Build history of the part. All positions in model axes, mm. Face numbers are marked on the shaded views. A direction names the side the tool comes from. Give positions to 0.01 mm unless a question says otherwise; leave off trailing zeros. Order: outer loops, then holes, each group sorted by start corner. A loop starts at its lowest first (then second) coordinate and runs counter-clockwise, first axis right, second up. Notation, with made-up numbers: (1, 46) -> (23, 46) arc R27 ccw to (23, 76) -> close; hole circle Ø3 at (85.5, 47). An arc over 180 degrees is marked (long way). Use a Markdown table: item, result. Add a question column.
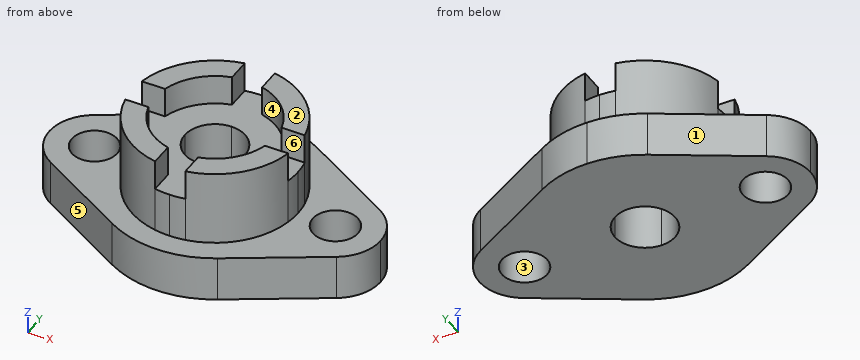
```python
from build123d import *

# Parameters (mm, degrees)
F1_DEPTH = 19.05
F2_DEPTH = 38.1
F3_DEPTH = 50.8


with BuildPart() as f1:
    # F0 (on Top) → F1 (new body)
    with BuildSketch(Plane.XY):
        with BuildLine():
            Line((41.275, 0), (34.925, 0))
            ThreePointArc((34.925, 0), (34.7791644937, -3.1883133656), (34.3428758988, -6.35))
            ThreePointArc((34.3428758988, -6.35), (24.6957043329, -24.6957043329), (6.35, -34.3428758988))
            ThreePointArc((6.35, -34.3428758988), (3.1883133656, -34.7791644937), (0, -34.925))
            ThreePointArc((0, -34.925), (-3.1883133656, -34.7791644937), (-6.35, -34.3428758988))
            ThreePointArc((-6.35, -34.3428758988), (-24.6957043329, -24.6957043329), (-34.3428758988, -6.35))
            ThreePointArc((-34.3428758988, -6.35), (-34.7791644937, -3.1883133656), (-34.925, 0))
            ThreePointArc((-34.925, 0), (-34.7791644937, 3.1883133656), (-34.3428758988, 6.35))
            ThreePointArc((-34.3428758988, 6.35), (-24.6957043329, 24.6957043329), (-6.35, 34.3428758988))
            ThreePointArc((-6.35, 34.3428758988), (-3.1883133656, 34.7791644937), (0, 34.925))
            Line((0, 34.925), (0, 44.45))
            ThreePointArc((0, 44.45), (-11.5045065548, 42.9354029785), (-22.225, 38.4948291982))
            Line((-22.225, 38.4948291982), (-60.325, 16.4977839421))
            ThreePointArc((-60.325, 16.4977839421), (-67.2977839421, 9.525), (-69.85, 0))
            ThreePointArc((-69.85, 0), (-67.2977839421, -9.525), (-60.325, -16.4977839421))
            Line((-60.325, -16.4977839421), (-22.225, -38.4948291982))
            ThreePointArc((-22.225, -38.4948291982), (0, -44.45), (22.225, -38.4948291982))
            Line((22.225, -38.4948291982), (60.325, -16.4977839421))
            ThreePointArc((60.325, -16.4977839421), (67.2977839421, -9.525), (69.85, 0))
            Line((69.85, 0), (60.325, 0))
            ThreePointArc((60.325, 0), (50.8, -9.525), (41.275, 0))
        make_face()
        with BuildLine():
            ThreePointArc((-41.275, 0), (-50.8, -9.525), (-60.325, 0))
            ThreePointArc((-60.325, 0), (-50.8, 9.525), (-41.275, 0))
        make_face(mode=Mode.SUBTRACT)
        with BuildLine():
            ThreePointArc((34.3428758988, 6.35), (34.7791644937, 3.1883133656), (34.925, 0))
            Line((34.925, 0), (41.275, 0))
            ThreePointArc((41.275, 0), (50.8, 9.525), (60.325, 0))
            Line((60.325, 0), (69.85, 0))
            ThreePointArc((69.85, 0), (67.2977839421, 9.525), (60.325, 16.4977839421))
            Line((60.325, 16.4977839421), (22.225, 38.4948291982))
            ThreePointArc((22.225, 38.4948291982), (11.5045065548, 42.9354029785), (0, 44.45))
            Line((0, 44.45), (0, 34.925))
            ThreePointArc((0, 34.925), (3.1883133656, 34.7791644937), (6.35, 34.3428758988))
            ThreePointArc((6.35, 34.3428758988), (24.6957043329, 24.6957043329), (34.3428758988, 6.35))
        make_face()
    extrude(amount=F1_DEPTH)

    # F0 (on Top) → F2 (join)
    with BuildSketch(Plane.XY):
        with BuildLine():
            Line((-6.35, -34.3428758988), (-6.35, -24.5934442484))
            ThreePointArc((-6.35, -24.5934442484), (-17.9605122421, -17.9605122421), (-24.5934442484, -6.35))
            Line((-24.5934442484, -6.35), (-34.3428758988, -6.35))
            ThreePointArc((-34.3428758988, -6.35), (-24.6957043329, -24.6957043329), (-6.35, -34.3428758988))
        make_face()
        with BuildLine():
            ThreePointArc((-24.5934442484, -6.35), (-25.1975542852, -3.2005090291), (-25.4, 0))
            Line((-25.4, 0), (-34.925, 0))
            ThreePointArc((-34.925, 0), (-34.7791644937, -3.1883133656), (-34.3428758988, -6.35))
            Line((-34.3428758988, -6.35), (-24.5934442484, -6.35))
        make_face()
        with BuildLine():
            Line((-34.925, 0), (-25.4, 0))
            ThreePointArc((-25.4, 0), (-25.1975542852, 3.2005090291), (-24.5934442484, 6.35))
            Line((-24.5934442484, 6.35), (-34.3428758988, 6.35))
            ThreePointArc((-34.3428758988, 6.35), (-34.7791644937, 3.1883133656), (-34.925, 0))
        make_face()
        with BuildLine():
            ThreePointArc((-24.5934442484, 6.35), (-17.9605122421, 17.9605122421), (-6.35, 24.5934442484))
            Line((-6.35, 24.5934442484), (-6.35, 34.3428758988))
            ThreePointArc((-6.35, 34.3428758988), (-24.6957043329, 24.6957043329), (-34.3428758988, 6.35))
            Line((-34.3428758988, 6.35), (-24.5934442484, 6.35))
        make_face()
        with BuildLine():
            ThreePointArc((-6.35, 24.5934442484), (-3.2005090291, 25.1975542852), (0, 25.4))
            Line((0, 25.4), (0, 34.925))
            ThreePointArc((0, 34.925), (-3.1883133656, 34.7791644937), (-6.35, 34.3428758988))
            Line((-6.35, 34.3428758988), (-6.35, 24.5934442484))
        make_face()
        with BuildLine():
            Line((0, 34.925), (0, 25.4))
            ThreePointArc((0, 25.4), (3.2005090291, 25.1975542852), (6.35, 24.5934442484))
            Line((6.35, 24.5934442484), (6.35, 34.3428758988))
            ThreePointArc((6.35, 34.3428758988), (3.1883133656, 34.7791644937), (0, 34.925))
        make_face()
        with BuildLine():
            ThreePointArc((6.35, 24.5934442484), (17.9605122421, 17.9605122421), (24.5934442484, 6.35))
            Line((24.5934442484, 6.35), (34.3428758988, 6.35))
            ThreePointArc((34.3428758988, 6.35), (24.6957043329, 24.6957043329), (6.35, 34.3428758988))
            Line((6.35, 34.3428758988), (6.35, 24.5934442484))
        make_face()
        with BuildLine():
            ThreePointArc((24.5934442484, 6.35), (25.1975542852, 3.2005090291), (25.4, 0))
            Line((25.4, 0), (34.925, 0))
            ThreePointArc((34.925, 0), (34.7791644937, 3.1883133656), (34.3428758988, 6.35))
            Line((34.3428758988, 6.35), (24.5934442484, 6.35))
        make_face()
        with BuildLine():
            ThreePointArc((6.35, -24.5934442484), (3.2005090291, -25.1975542852), (0, -25.4))
            Line((0, -25.4), (0, -34.925))
            ThreePointArc((0, -34.925), (3.1883133656, -34.7791644937), (6.35, -34.3428758988))
            Line((6.35, -34.3428758988), (6.35, -24.5934442484))
        make_face()
        with BuildLine():
            Line((0, -34.925), (0, -25.4))
            ThreePointArc((0, -25.4), (-3.2005090291, -25.1975542852), (-6.35, -24.5934442484))
            Line((-6.35, -24.5934442484), (-6.35, -34.3428758988))
            ThreePointArc((-6.35, -34.3428758988), (-3.1883133656, -34.7791644937), (0, -34.925))
        make_face()
        with BuildLine():
            Line((34.925, 0), (25.4, 0))
            ThreePointArc((25.4, 0), (25.1975542852, -3.2005090291), (24.5934442484, -6.35))
            Line((24.5934442484, -6.35), (34.3428758988, -6.35))
            ThreePointArc((34.3428758988, -6.35), (34.7791644937, -3.1883133656), (34.925, 0))
        make_face()
        with BuildLine():
            Line((34.3428758988, -6.35), (24.5934442484, -6.35))
            ThreePointArc((24.5934442484, -6.35), (17.9605122421, -17.9605122421), (6.35, -24.5934442484))
            Line((6.35, -24.5934442484), (6.35, -34.3428758988))
            ThreePointArc((6.35, -34.3428758988), (24.6957043329, -24.6957043329), (34.3428758988, -6.35))
        make_face()
        with BuildLine():
            Line((0, -25.4), (0, -12.7))
            ThreePointArc((0, -12.7), (-8.9802561211, -8.9802561211), (-12.7, 0))
            Line((-12.7, 0), (-25.4, 0))
            ThreePointArc((-25.4, 0), (-25.1975542852, -3.2005090291), (-24.5934442484, -6.35))
            ThreePointArc((-24.5934442484, -6.35), (-17.9605122421, -17.9605122421), (-6.35, -24.5934442484))
            ThreePointArc((-6.35, -24.5934442484), (-3.2005090291, -25.1975542852), (0, -25.4))
        make_face()
        with BuildLine():
            Line((25.4, 0), (12.7, 0))
            ThreePointArc((12.7, 0), (8.9802561211, -8.9802561211), (0, -12.7))
            Line((0, -12.7), (0, -25.4))
            ThreePointArc((0, -25.4), (3.2005090291, -25.1975542852), (6.35, -24.5934442484))
            ThreePointArc((6.35, -24.5934442484), (17.9605122421, -17.9605122421), (24.5934442484, -6.35))
            ThreePointArc((24.5934442484, -6.35), (25.1975542852, -3.2005090291), (25.4, 0))
        make_face()
        with BuildLine():
            ThreePointArc((0, 12.7), (8.9802561211, 8.9802561211), (12.7, 0))
            Line((12.7, 0), (25.4, 0))
            ThreePointArc((25.4, 0), (25.1975542852, 3.2005090291), (24.5934442484, 6.35))
            ThreePointArc((24.5934442484, 6.35), (17.9605122421, 17.9605122421), (6.35, 24.5934442484))
            ThreePointArc((6.35, 24.5934442484), (3.2005090291, 25.1975542852), (0, 25.4))
            Line((0, 25.4), (0, 12.7))
        make_face()
        with BuildLine():
            ThreePointArc((-12.7, 0), (-8.9802561211, 8.9802561211), (0, 12.7))
            Line((0, 12.7), (0, 25.4))
            ThreePointArc((0, 25.4), (-3.2005090291, 25.1975542852), (-6.35, 24.5934442484))
            ThreePointArc((-6.35, 24.5934442484), (-17.9605122421, 17.9605122421), (-24.5934442484, 6.35))
            ThreePointArc((-24.5934442484, 6.35), (-25.1975542852, 3.2005090291), (-25.4, 0))
            Line((-25.4, 0), (-12.7, 0))
        make_face()
    extrude(amount=F2_DEPTH)

    # F0 (on Top) → F3 (join)
    with BuildSketch(Plane.XY):
        with BuildLine():
            Line((-6.35, -34.3428758988), (-6.35, -24.5934442484))
            ThreePointArc((-6.35, -24.5934442484), (-17.9605122421, -17.9605122421), (-24.5934442484, -6.35))
            Line((-24.5934442484, -6.35), (-34.3428758988, -6.35))
            ThreePointArc((-34.3428758988, -6.35), (-24.6957043329, -24.6957043329), (-6.35, -34.3428758988))
        make_face()
        with BuildLine():
            Line((34.3428758988, -6.35), (24.5934442484, -6.35))
            ThreePointArc((24.5934442484, -6.35), (17.9605122421, -17.9605122421), (6.35, -24.5934442484))
            Line((6.35, -24.5934442484), (6.35, -34.3428758988))
            ThreePointArc((6.35, -34.3428758988), (24.6957043329, -24.6957043329), (34.3428758988, -6.35))
        make_face()
        with BuildLine():
            ThreePointArc((6.35, 24.5934442484), (17.9605122421, 17.9605122421), (24.5934442484, 6.35))
            Line((24.5934442484, 6.35), (34.3428758988, 6.35))
            ThreePointArc((34.3428758988, 6.35), (24.6957043329, 24.6957043329), (6.35, 34.3428758988))
            Line((6.35, 34.3428758988), (6.35, 24.5934442484))
        make_face()
        with BuildLine():
            ThreePointArc((-24.5934442484, 6.35), (-17.9605122421, 17.9605122421), (-6.35, 24.5934442484))
            Line((-6.35, 24.5934442484), (-6.35, 34.3428758988))
            ThreePointArc((-6.35, 34.3428758988), (-24.6957043329, 24.6957043329), (-34.3428758988, 6.35))
            Line((-34.3428758988, 6.35), (-24.5934442484, 6.35))
        make_face()
    extrude(amount=F3_DEPTH)


solid = f1.part
```
(1) Band-saw the part on D-D on x = 31.5. Give the cut face in (y, z).
(2) Mould opens along Y. For the marked faces 1, 2 and 3 say: released by +Y, released by -Y, zero draft, split by the parting line, or undercut.
(3) Band-saw the part on A-A on z = 5. Give the cut face in (x, y) (3 decimals).
(4) Tool access for the marked faces 4, 5 and 6: list every direction of +Z, -Z, +X, -X, +Y, -Y with a clear straight run to the whole face (end or side of a thin tool).
(5) Band-saw the part on C-C on y = -32.5. Give the cut face in (x, z), plus the area to 3 significant figures.
(6) Wall check: probe 1 along X at (y, z) = (7.5, 11.5); probe 2 along Y at (x, z) = (13.5, 41); probe 3 along Z at (x, y) = (18.5, -38). Give the ranges that are in metal, low to high.
(7) Pin check, flat tips, straight feed: pin 1 Ø8 at (y, z) = (32, 41.5) entering from -X; pin 2 Ø6 at (x, z) = (-25, 6) entering from -Y; pin 3 Ø3 at (x, z) = (-30.5, 46) entering from +Y. Stop position of each tip, or through.
(8) Band-saw the part on B-B on x = -50.8. Give the cut face in (y, z) (3 decimals), plus the area to 3 significant figures.
Response:
| question | item | result |
|---|---|---|
| 1 | outline | (-33.14, 0) -> (33.14, 0) -> (33.14, 19.05) -> (15.08, 19.05) -> (15.08, 50.8) -> (6.35, 50.8) -> (6.35, 38.1) -> (-6.35, 38.1) -> (-6.35, 50.8) -> (-15.08, 50.8) -> (-15.08, 19.05) -> (-33.14, 19.05) -> close |
| 2 | face 1 | released by +Y |
| 2 | face 2 | zero draft |
| 2 | face 3 | undercut |
| 3 | outline | (-60.325, -16.498) -> (-22.225, -38.495) arc R44.45 ccw to (22.225, -38.495) -> (60.325, -16.498) arc R19.05 ccw to (60.325, 16.498) -> (22.225, 38.495) arc R44.45 ccw to (-22.225, 38.495) -> (-60.325, 16.498) arc R19.05 ccw to start; hole circle Ø19.05 at (-50.8, 0); hole circle Ø25.4 at (0, 0); hole circle Ø19.05 at (50.8, 0) |
| 4 | face 4 | +Z |
| 4 | face 5 | +Z, -Z, -X, -Y |
| 4 | face 6 | +Z, +X, -X |
| 5 | outline | (-32.61, 0) -> (32.61, 0) -> (32.61, 19.05) -> (12.79, 19.05) -> (12.79, 50.8) -> (6.35, 50.8) -> (6.35, 38.1) -> (-6.35, 38.1) -> (-6.35, 50.8) -> (-12.79, 50.8) -> (-12.79, 19.05) -> (-32.61, 19.05) -> close |
| 5 | area | 1,890 mm² |
| 6 | probe 1 | x = -68.31 to -56.67, -44.93 to -10.25, 10.25 to 44.93, 56.67 to 68.31 |
| 6 | probe 2 | y = -32.21 to -21.52, 21.52 to 32.21 |
| 6 | probe 3 | z = 0 to 19.05 |
| 7 | pin 1 | stops at x = -20.87 |
| 7 | pin 2 | stops at y = -38.62 |
| 7 | pin 3 | stops at y = 19.46 |
| 8 | outline | (-21.997, 0) -> (-9.525, 0) -> (-9.525, 19.05) -> (-21.997, 19.05) -> close; (9.525, 0) -> (21.997, 0) -> (21.997, 19.05) -> (9.525, 19.05) -> close |
| 8 | area | 475 mm² |
